```python
from build123d import *

# Parameters (mm, degrees)
SKETCH1_W                 = 32
SKETCH1_H                 = 65
BOSS_EXTRUDE1_DEPTH       = 32
SHELL1_T                  = -2.5
SHELL1_THICKNESS_2_FACE_W = 60
SHELL1_THICKNESS_2_FACE_H = 27
SHELL1_THICKNESS_2_DEPTH  = 15
SHELL2_START              = 2.5
SHELL2_OUTLINE_W          = 15
SHELL2_OUTLINE_H          = 60
SHELL2_DEPTH              = 27
SKETCH2_R                 = 4
BOSS_EXTRUDE2_DEPTH       = 2


# Read off the part's stored shape, not the designer's step: Shell2
with BuildPart() as part:
    # Sketch1 → Boss-Extrude1 (new body)
    with BuildSketch(Plane(origin=(0, 0, 0), x_dir=(1, 0, 0), z_dir=(0, 1, 0))):
        with Locations((16, -32.5)):
            Rectangle(SKETCH1_W, SKETCH1_H)
    extrude(amount=BOSS_EXTRUDE1_DEPTH)

    # Shell1
    shell1_openings = [part.faces().sort_by_distance(p)[0] for p in [
        (16, 32, 32.5),
    ]]
    offset(amount=SHELL1_T, openings=shell1_openings, kind=Kind.INTERSECTION)

    # Shell1 thickness 2 face (on inner face of the shell) → Shell1 thickness 2 (add)
    with BuildSketch(Plane(origin=(16, 2.5, 32.5), x_dir=(0, 0, -1), z_dir=(0, -1, 0))):
        Rectangle(SHELL1_THICKNESS_2_FACE_W, SHELL1_THICKNESS_2_FACE_H)
    extrude(amount=-SHELL1_THICKNESS_2_DEPTH)

    # Shell2 outline → Shell2 (cut)
    with BuildSketch(Plane.YZ.offset(SHELL2_START)):
        with Locations((7.5, 32.5)):
            Rectangle(SHELL2_OUTLINE_W, SHELL2_OUTLINE_H)
    extrude(amount=SHELL2_DEPTH, mode=Mode.SUBTRACT)

    # Sketch2 → Boss-Extrude2 (add)
    with BuildSketch(Plane.XY.offset(65)):
        with Locations(Location((7.5, 24.5, 0), (0, 0, 180))):
            Circle(SKETCH2_R)
        with Locations(Location((19.5, 24.5, 0), (0, 0, 180))):
            Circle(SKETCH2_R)
    extrude(amount=BOSS_EXTRUDE2_DEPTH)


solid = part.part
```
Here's how the part is built. I have some questions about the finished solid (model axes, mm). A direction names the side the tool comes from. Coordinates: 2 decimals unless noted, no trailing zeros. Write each loop counter-clockwise with the first axis right and the second up, starting at its lowest first coordinate (ties: lowest second). Pieces come first, ordered by that corner, then holes. Notation, with made-up numbers: (12.5, 73) -> (23.5, 73) arc R12 cw to (23.5, 95) -> close; hole circle Ø9 at (54.5, 46). An arc over 180 degrees is marked (long way). Use a Markdown table: item, result. Add a question column.
(1) If we section it at B-B, the plane x = 7.5: Write out the boundary of the cut face in (y, z), and give its area (3 significant figures).
(2) If we section it at A-A, the plane y = 24.5: Write out the boundary of the cut face in (x, z), and give its area (3 significant figures).
(3) If we section it at D-D, the plane y = 5.5: Write out the boundary of the cut face in (x, z), and give its area (3 significant figures).
(4) For faces 1 (the cylindrical face through (20.021, 20.534, 65.986)), 2 (the flat face through (16, 15, 32)), 3 (the flat face through (16, 17.5, 33)), which set-ups out of +Z, -Z, +X, -X, +Y, -Y let a thin tool reach every point of the face, with its end or its side?
(5) If we section it at C-C, the plane z = 44: Write out the boundary of the cut face in (x, y), and give its area (4 significant figures).
(6) We'd pull the mould along X, two halves only. Please class faces 4 (the flat face through (32, 16, 33)), 5 (the flat face through (20, 24, 67)), 6 (the flat face through (29.5, 7, 33)): +X half, -X half, draft (parallel to the pull), parting line (faces both ways), or undercut.
(7) I'm going to push flat-ended pins straight in: P1, Ø4.5, axis at x = 13, y = 5, coming from the -Z side; P2, Ø2, axis at x = 23, z = 31.5, coming from the +Y side; P3, Ø16.5, axis at x = 21.5, y = 8.5, coming from the +Z side; P4, Ø1, axis at x = 4, z = 52, coming from the -Y side. Where does each tip first touch, or does it pass through?
(8) Please list where these lines run through material, in increasing order: line 1 (Z direction, x = 6.5, y = 12.5); line 2 (X direction, y = 10, z = 45.5); line 3 (Y direction, x = 11, z = 36).
Outcome:
| question | item | result |
|---|---|---|
| 1 | outline | (0, 0) -> (32, 0) -> (32, 2.5) -> (17.5, 2.5) -> (17.5, 62.5) -> (32, 62.5) -> (32, 65) -> (28.5, 65) -> (28.5, 67) -> (20.5, 67) -> (20.5, 65) -> (0, 65) -> (0, 62.5) -> (15, 62.5) -> (15, 2.5) -> (0, 2.5) -> close |
| 1 | area | 326 mm^2 |
| 2 | outline | (0, 0) -> (32, 0) -> (32, 65) -> (23.5, 65) -> (23.5, 67) -> (15.5, 67) -> (15.5, 65) -> (11.5, 65) -> (11.5, 67) -> (3.5, 67) -> (3.5, 65) -> (0, 65) -> close; hole (2.5, 2.5) -> (29.5, 2.5) -> (29.5, 62.5) -> (2.5, 62.5) -> close |
| 2 | area | 492 mm^2 |
| 3 | outline | (0, 0) -> (32, 0) -> (32, 65) -> (0, 65) -> close; hole (2.5, 2.5) -> (29.5, 2.5) -> (29.5, 62.5) -> (2.5, 62.5) -> close |
| 3 | area | 460 mm^2 |
| 4 | face 1 | +Z |
| 4 | face 2 | -Y |
| 4 | face 3 | +Y |
| 5 | outline | (0, 0) -> (2.5, 0) -> (2.5, 15) -> (29.5, 15) -> (29.5, 0) -> (32, 0) -> (32, 32) -> (29.5, 32) -> (29.5, 17.5) -> (2.5, 17.5) -> (2.5, 32) -> (0, 32) -> close |
| 5 | area | 227.5 mm^2 |
| 6 | face 4 | +X half |
| 6 | face 5 | draft |
| 6 | face 6 | undercut |
| 7 | P1 | stops at z = 0 |
| 7 | P2 | stops at y = 17.5 |
| 7 | P3 | stops at z = 65 |
| 7 | P4 | stops at y = 15 |
| 8 | line 1 | z = 0 to 2.5, 62.5 to 65 |
| 8 | line 2 | x = 0 to 2.5, 29.5 to 32 |
| 8 | line 3 | y = 15 to 17.5 |
